For this review, take the finished solid that the model builds, in its own axes (mm). Face numbers are marked on the shaded views. A direction names the side the tool comes from. Coordinates: 2 decimals unless noted, no trailing zeros. Write each loop counter-clockwise with the first axis right and the second up, starting at its lowest first coordinate (ties: lowest second). Pieces come first, ordered by that corner, then holes.
1) We need section D-D on z = 9. Write out the cut boundary in (x, y), then the cut area to 3 significant figures.
2) For the marked faces 1 and 2, list the 3-axis set-ups (+Z, -Z, +X, -X, +Y, -Y) from which the entire face can be reached by the end or side of a thin tool; tool diameter is ignored.
3) To check wall thickness, follow line 1 along Y through (x, z) = (0, -2.5); line 2 along Y through (x, z) = (-21, -4); line 3 along X through (y, z) = (74, -1). State the ranges of each line that lie inside material, in increasing order.
4) We need section C-C on y = 67.12. Write out the cut boundary in (x, z) (1 decimal).
5) We need section A-A on x = 0. Write out the cut boundary in (y, z), then the cut area to 3 significant figures.
6) Insertion check: P1, Ø2.5, axis at x = 16.36, z = -2.15, coming from the +Y side; P2, Ø10, axis at x = -11, z = 2, coming from the -Y side; P3, Ø3.5, axis at x = 0, y = 74.12, coming from the +Z side; P4, Ø12, axis at x = -13, z = -2, coming from the +Y side. Each pin has a flat end and moves straight along its axis. Give the tip position at first contact, or say it passes through.
7) We need section B-B on z = 15.5. Write out the cut boundary in (x, y), then the cut area to 3 significant figures.
from build123d import *

# Parameters (mm, degrees)
SKETCH1_R               = 26.65
BOSS_EXTRUDE1_DEPTH     = 2.54
SKETCH2_R               = 12.7
BOSS_EXTRUDE2_DEPTH     = 5.08
SKETCH4_R               = 4.7625
BOSS_EXTRUDE3_DEPTH     = 70
SKETCH6_R               = 1.5
CUT_EXTRUDE2_DEPTH      = 87.286206314
CUT_EXTRUDE3_DEPTH      = 87.286206314
CUT_EXTRUDE3_DEPTH_BACK = 87.286206314
SKETCH7_R               = 1.5
CUT_EXTRUDE4_DEPTH      = 87.286206404
CUT_EXTRUDE4_DEPTH_BACK = 87.286206404
SKETCH8_R               = 1.5


with BuildPart() as part:
    # Sketch1 → Boss-Extrude1 (new body)
    with BuildSketch(Plane(origin=(0, 0, 0), x_dir=(1, 0, 0), z_dir=(0, 1, 0))):
        with Locations(Location((0, 0, 0), (0, 0, 270))):
            Circle(SKETCH1_R)
    extrude(amount=BOSS_EXTRUDE1_DEPTH)

    # Sketch2 → Boss-Extrude2 (add)
    with BuildSketch(Plane(origin=(0, 2.54, 0), x_dir=(1, 0, 0), z_dir=(0, 1, 0))):
        with Locations(Location((0, 0, 0), (0, 0, 270))):
            Circle(SKETCH2_R)
    extrude(amount=BOSS_EXTRUDE2_DEPTH)

    # Sketch4 → Boss-Extrude3 (add)
    with BuildSketch(Plane(origin=(0, 7.62, 0), x_dir=(1, 0, 0), z_dir=(0, 1, 0))):
        with Locations(Location((0, 0, 0), (0, 0, 270))):
            Circle(SKETCH4_R)
    extrude(amount=BOSS_EXTRUDE3_DEPTH)

    # Sketch6 → Cut-Extrude2 (cut, through all)
    with BuildSketch(Plane(origin=(0, 0, 0), x_dir=(-1, 0, 0), z_dir=(0, -1, 0))):
        with Locations(Location((6.313805851, -15.242875716, 0), (0, 0, 90))):
            Circle(SKETCH6_R)
        with Locations(Location((-16.357620523, 2.153521596, 0), (0, 0, 90))):
            Circle(SKETCH6_R)
        with Locations(Location((10.043814672, 13.08935412, 0), (0, 0, 90))):
            Circle(SKETCH6_R)
        with Locations(Location((-3.403504282, -19.302231959, 0), (0, 0, 90))):
            Circle(SKETCH6_R)
        with Locations(Location((-18.417975367, 6.703594809, 0), (0, 0, 90))):
            Circle(SKETCH6_R)
        with Locations(Location((-15.014471085, 12.59863715, 0), (0, 0, 90))):
            Circle(SKETCH6_R)
        with Locations(Location((15.014471085, 12.59863715, 0), (0, 0, 90))):
            Circle(SKETCH6_R)
        with Locations(Location((18.417975367, 6.703594809, 0), (0, 0, 90))):
            Circle(SKETCH6_R)
        with Locations(Location((3.403504282, -19.302231959, 0), (0, 0, 90))):
            Circle(SKETCH6_R)
    extrude(amount=-CUT_EXTRUDE2_DEPTH, mode=Mode.SUBTRACT)

    # Sketch7 → Cut-Extrude3 (cut, two sides: drawn at the far end of the back side and taken through both)
    with BuildSketch(Plane.XY.offset(-CUT_EXTRUDE3_DEPTH_BACK)):
        with Locations(Location((0, 74.12, 0), (0, 0, 90.00000001))):
            Circle(SKETCH7_R)
    extrude(amount=CUT_EXTRUDE3_DEPTH + CUT_EXTRUDE3_DEPTH_BACK, mode=Mode.SUBTRACT)

    # Sketch8 → Cut-Extrude4 (cut, two sides: drawn at the far end of the back side and taken through both)
    with BuildSketch(Plane(origin=(0, 0, 0), x_dir=(0, 0, -1), z_dir=(1, 0, 0)).offset(-CUT_EXTRUDE4_DEPTH_BACK)):
        with Locations((0, 67.12)):
            Circle(SKETCH8_R)
    extrude(amount=CUT_EXTRUDE4_DEPTH + CUT_EXTRUDE4_DEPTH_BACK, mode=Mode.SUBTRACT)


solid = part.part
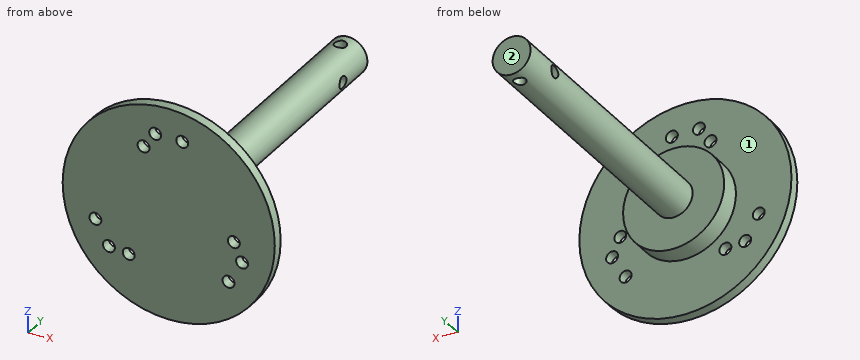
Result:
1. outline: (-25.08, 0) - (25.08, 0) - (25.08, 2.54) - (8.96, 2.54) - (8.96, 7.62) - (-8.96, 7.62) - (-8.96, 2.54) - (-25.08, 2.54) - close
1. area: 218 mm2
2. face 1: +Y
2. face 2: +Z, -Z, +X, -X, +Y
3. line 1: y = 0 to 72.62, 75.62 to 77.62
3. line 2: y = 0 to 2.54
3. line 3: x = -4.66 to -1.5, 1.5 to 4.66
4. outline: (-4.5, -1.5) arc R4.8 ccw to (4.5, -1.5) - close; (-4.5, 1.5) - (4.5, 1.5) arc R4.8 ccw to start
5. outline: (0, -26.65) - (2.54, -26.65) - (2.54, -12.7) - (7.62, -12.7) - (7.62, -4.76) - (72.62, -4.76) - (72.62, 4.76) - (7.62, 4.76) - (7.62, 12.7) - (2.54, 12.7) - (2.54, 26.65) - (0, 26.65) - close; (75.62, -4.76) - (77.62, -4.76) - (77.62, 4.76) - (75.62, 4.76) - close; hole circle Ø3 at (67.12, 0)
5. area: 896 mm2
6. P1: passes through
6. P2: stops at y = 0
6. P3: stops at z = 4.76
6. P4: stops at y = 7.62
7. outline: (-21.68, 0) - (-7.79, 0) - (-7.79, 2.54) - (-21.68, 2.54) - close; (-4.84, 0) - (21.68, 0) - (21.68, 2.54) - (-4.84, 2.54) - close
7. area: 103 mm2
